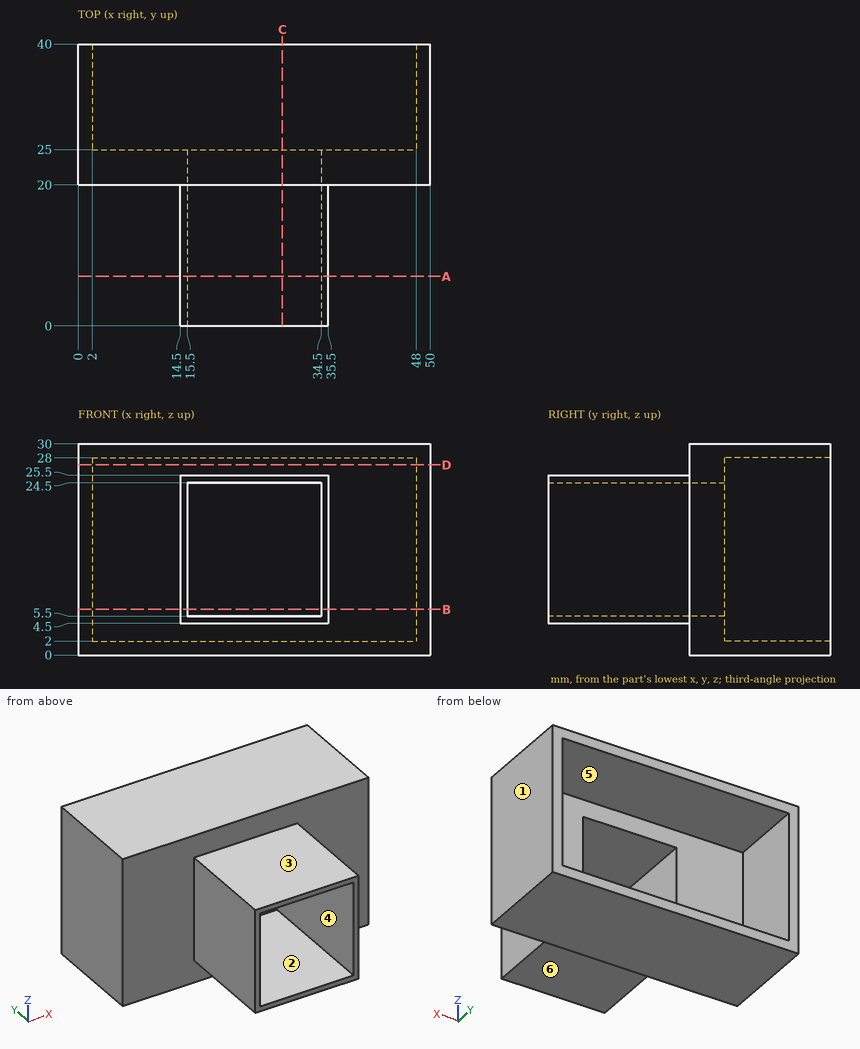
Here's the drawing with two shaded views (mm, measured from the low corner). I have some questions. A direction names the side the tool comes from. Give positions to 0.01 mm unless a question says otherwise; leave off trailing zeros. Order: outer loops, then holes, each group sorted by start corner. A loop starts at its lowest first (then second) coordinate and runs counter-clockwise, first axis right, second up. Notation, with made-up numbers: (52, 48.25) -> (89, 48.25) arc R22 cw to (89, 57.25) -> close; hole circle Ø5 at (44.25, 85). An arc over 180 degrees is marked (long way). Use a Markdown table: item, result. Add a question column.
Item 1: Imagine slicing it at C-C on x = 29. Please give me the cut outline in (y, z).
Item 2: Will these pins go through, and if not, where does the flat tip stop? pin 1 (7.5 mm diameter, centred on y = 35.5, z = 13, fed in from -X); pin 2 (9.5 mm diameter, centred on x = 28, y = 9, fed in from +Z); pin 3 (4 mm diameter, centred on x = 17, z = 16.5, fed in from +Y); pin 4 (16 mm diameter, centred on y = 10.5, z = 14, fed in from +X).
Item 3: Imagine slicing it at A-A on y = 7. Please give me the cut outline in (x, z), plus the area to 3 significant figures.
Item 4: I need wall thicknesses on line 1 (Z direction, x = 28, y = 4); line 2 (Z direction, x = 38.5, y = 27); line 3 (X direction, y = 13, z = 9.5). Which ranges of each line are inside material? Lowest first, please.
Item 5: Imagine slicing it at B-B on z = 6.5. Please give me the cut outline in (x, y), plus the area to 3 significant figures.
Item 6: For the marked faces 4, 5 and 6, which set-ups out of +Z, -Z, +X, -X, +Y, -Y let a thin tool reach every point of the face, with its end or its side?
Item 7: Imagine slicing it at D-D on z = 27. Please give me the cut outline in (x, y), plus the area to 3 significant figures.
Item 8: If we mould it in two halves opening along X, with no side actions, what happens to the marked faces 1, 2 and 3? For each: pulls with the +X half, pulls with the -X half, needs draft (parallel to the pull), parting line crosses it, or undercut.
Data:
| question | item | result |
|---|---|---|
| 1 | outline | (0, 4.5) -> (20, 4.5) -> (20, 0) -> (40, 0) -> (40, 2) -> (25, 2) -> (25, 5.5) -> (0, 5.5) -> close; (0, 24.5) -> (25, 24.5) -> (25, 28) -> (40, 28) -> (40, 30) -> (20, 30) -> (20, 25.5) -> (0, 25.5) -> close |
| 2 | pin 1 | stops at x = 0 |
| 2 | pin 2 | stops at z = 25.5 |
| 2 | pin 3 | stops at y = 25 |
| 2 | pin 4 | stops at x = 35.5 |
| 3 | outline | (14.5, 4.5) -> (35.5, 4.5) -> (35.5, 25.5) -> (14.5, 25.5) -> close; hole (15.5, 5.5) -> (34.5, 5.5) -> (34.5, 24.5) -> (15.5, 24.5) -> close |
| 3 | area | 80.0 mm² |
| 4 | line 1 | z = 4.5 to 5.5, 24.5 to 25.5 |
| 4 | line 2 | z = 0 to 2, 28 to 30 |
| 4 | line 3 | x = 14.5 to 15.5, 34.5 to 35.5 |
| 5 | outline | (0, 20) -> (14.5, 20) -> (14.5, 0) -> (15.5, 0) -> (15.5, 25) -> (2, 25) -> (2, 40) -> (0, 40) -> close; (34.5, 0) -> (35.5, 0) -> (35.5, 20) -> (50, 20) -> (50, 40) -> (48, 40) -> (48, 25) -> (34.5, 25) -> close |
| 5 | area | 255 mm² |
| 6 | face 4 | +Y, -Y |
| 6 | face 5 | +Y |
| 6 | face 6 | -Z, +X, -X, -Y |
| 7 | outline | (0, 20) -> (50, 20) -> (50, 40) -> (48, 40) -> (48, 25) -> (2, 25) -> (2, 40) -> (0, 40) -> close |
| 7 | area | 310 mm² |
| 8 | face 1 | pulls with the +X half |
| 8 | face 2 | undercut |
| 8 | face 3 | needs draft |
